```python
from build123d import *

# Parameters (mm, degrees)
EXTRUDE_1_DEPTH      = 20
EXTRUDE_1_DEPTH_BACK = 20
SKETCH_1_W           = 140
SKETCH_1_H           = 580
SKETCH_1_R           = 30
EXTRUDE_2_DEPTH      = 25
EXTRUDE_2_DEPTH_BACK = 65
SKETCH_3_R           = 30
CUT_EXTRUDE_1_DEPTH  = 40
FILLET_1_R           = 50
FILLET_2_R           = 15
CHAMFER_1_SIZE       = 20


with BuildPart() as part:
    # Эскиз1 → Бобышка-Вытянуть1 (new, two sides: drawn at the far end of the back side and taken through both)
    with BuildSketch(Plane.XY.offset(-EXTRUDE_1_DEPTH_BACK)):
        with Locations((0, -208.783389553)):
            Rectangle(SKETCH_1_W, SKETCH_1_H)
        with Locations((0, 41.216610447)):
            Circle(SKETCH_1_R, mode=Mode.SUBTRACT)
        with Locations((0, -458.783389553)):
            Circle(SKETCH_1_R, mode=Mode.SUBTRACT)
    extrude(amount=EXTRUDE_1_DEPTH + EXTRUDE_1_DEPTH_BACK)

    # Эскиз3 → Бобышка-Вытянуть2 (add, two sides: drawn at the far end of the back side and taken through both)
    with BuildSketch(Plane(origin=(0, 0, -20), x_dir=(-1, 0, 0), z_dir=(0, 0, -1)).offset(-EXTRUDE_2_DEPTH_BACK)):
        with Locations((0, 41.216610447)):
            Circle(SKETCH_3_R)
        with Locations((0, -458.783389553)):
            Circle(SKETCH_3_R)
    extrude(amount=EXTRUDE_2_DEPTH + EXTRUDE_2_DEPTH_BACK)

    # Эскиз4 → Вырез-Вытянуть1 (cut)
    with BuildSketch(Plane(origin=(0, 0, -20), x_dir=(-1, 0, 0), z_dir=(0, 0, -1))):
        Polygon((-30, 1.216610447), (0, 1.216610447), (30, 1.216610447), (30, -418.783389553), (0, -418.783389553), (-30, -418.783389553), align=None)
    extrude(amount=-CUT_EXTRUDE_1_DEPTH, mode=Mode.SUBTRACT)

    # Скругление1
    fillet_1_edges = [part.edges().sort_by_distance(p)[0] for p in [
        (70, -498.783389553, 0),
        (70, 81.216610447, 0),
        (-70, 81.216610447, 0),
        (-70, -498.783389553, 0),
    ]]
    fillet(fillet_1_edges, radius=FILLET_1_R)

    # Скругление2
    fillet_2_edges = [part.edges().sort_by_distance(p)[0] for p in [
        (30, 1.216610447, 0),
        (-30, 1.216610447, 0),
        (-30, -418.783389553, 0),
        (30, -418.783389553, 0),
    ]]
    fillet(fillet_2_edges, radius=FILLET_2_R)

    # Фаска1
    # the kernel refuses this chamfer: 20 mm, written as the material it takes off along each edge
    with BuildSketch(Plane(origin=(20, -498.783389553, -20), x_dir=(0, -0.0274958766105877, 0.9996219169112968), z_dir=(-1, 0, 0))) as chamfer_1_piece_1_section:
        Polygon((CHAMFER_1_SIZE * 0.999621916911, CHAMFER_1_SIZE * 0.0274958766106), (-CHAMFER_1_SIZE * 0.0274958766106, CHAMFER_1_SIZE * 0.999621916911), (0, 0), align=None)
    chamfer_1_piece_1 = extrude(amount=40, mode=Mode.PRIVATE)
    chamfer_1_piece_1 = chamfer_1_piece_1 - Plane(origin=(0, -458.783389553, -12.567480213), x_dir=(-1, 0, 0), z_dir=(0, 0, 1)) * Cylinder(30, 160, mode=Mode.PRIVATE)
    add(chamfer_1_piece_1, mode=Mode.SUBTRACT)
    with BuildSketch(Plane(origin=(-20, -448.783389553, -20), x_dir=(0, -1, 0), z_dir=(1, 0, 0))) as chamfer_1_piece_2_section:
        Polygon((50, -CHAMFER_1_SIZE), (50 - CHAMFER_1_SIZE, 0), (50, 0), align=None)
    chamfer_1_piece_2 = revolve(axis=Axis((-20, -448.783389553, -20), (0, 0, -1)), revolution_arc=90, mode=Mode.PRIVATE)
    chamfer_1_piece_2 = chamfer_1_piece_2 - Plane(origin=(0, -458.783389553, -13.088521936), x_dir=(-1, 0, 0), z_dir=(0, 0, 1)) * Cylinder(30, 200, mode=Mode.PRIVATE)
    add(chamfer_1_piece_2, mode=Mode.SUBTRACT)
    with BuildSketch(Plane(origin=(20, -448.783389553, -20), x_dir=(1, 0, 0), z_dir=(0, 1, 0))) as chamfer_1_piece_3_section:
        Polygon((50, -CHAMFER_1_SIZE), (50 - CHAMFER_1_SIZE, 0), (50, 0), align=None)
    chamfer_1_piece_3 = revolve(axis=Axis((20, -448.783389553, -20), (0, 0, -1)), revolution_arc=90, mode=Mode.PRIVATE)
    chamfer_1_piece_3 = chamfer_1_piece_3 - Plane(origin=(0, -458.783389553, -13.088521936), x_dir=(-1, 0, 0), z_dir=(0, 0, 1)) * Cylinder(30, 200, mode=Mode.PRIVATE)
    add(chamfer_1_piece_3, mode=Mode.SUBTRACT)
    with BuildSketch(Plane(origin=(-70, -448.783389553, -20), x_dir=(-0.027495876610586317, 0, 0.9996219169112968), z_dir=(0, 1, 0)), Plane(origin=(70, 31.216610447, -20), x_dir=(0.027495876610586317, 0, 0.9996219169112968), z_dir=(0, -1, 0)), Plane(origin=(70, 31.216610447, 20), x_dir=(-0.9996219169112968, 0, 0.027495876610586317), z_dir=(0, -1, 0)), Plane(origin=(-70, -448.783389553, 20), x_dir=(0.9996219169112968, 0, 0.027495876610586317), z_dir=(0, 1, 0))) as chamfer_1_piece_4:
        Polygon((CHAMFER_1_SIZE * 0.999621916911, CHAMFER_1_SIZE * 0.0274958766106), (-CHAMFER_1_SIZE * 0.0274958766106, CHAMFER_1_SIZE * 0.999621916911), (0, 0), align=None)
    extrude(amount=480, mode=Mode.SUBTRACT)
    with BuildSketch(Plane(origin=(-20, 31.216610447, -20), x_dir=(0, 1, 0), z_dir=(1, 0, 0))) as chamfer_1_piece_5_section:
        Polygon((50, CHAMFER_1_SIZE), (50 - CHAMFER_1_SIZE, 0), (50, 0), align=None)
    chamfer_1_piece_5 = revolve(axis=Axis((-20, 31.216610447, -20), (0, 0, 1)), revolution_arc=90, mode=Mode.PRIVATE)
    chamfer_1_piece_5 = chamfer_1_piece_5 - Plane(origin=(0, 41.216610447, -13.088521936), x_dir=(-1, 0, 0), z_dir=(0, 0, 1)) * Cylinder(30, 200, mode=Mode.PRIVATE)
    add(chamfer_1_piece_5, mode=Mode.SUBTRACT)
    with BuildSketch(Plane(origin=(20, 31.216610447, -20), x_dir=(1, 0, 0), z_dir=(0, -1, 0))) as chamfer_1_piece_6_section:
        Polygon((50, CHAMFER_1_SIZE), (50 - CHAMFER_1_SIZE, 0), (50, 0), align=None)
    chamfer_1_piece_6 = revolve(axis=Axis((20, 31.216610447, -20), (0, 0, 1)), revolution_arc=90, mode=Mode.PRIVATE)
    chamfer_1_piece_6 = chamfer_1_piece_6 - Plane(origin=(0, 41.216610447, -13.088521936), x_dir=(-1, 0, 0), z_dir=(0, 0, 1)) * Cylinder(30, 200, mode=Mode.PRIVATE)
    add(chamfer_1_piece_6, mode=Mode.SUBTRACT)
    with BuildSketch(Plane(origin=(-20, 81.216610447, -20), x_dir=(0, 0.027495876610586317, 0.9996219169112968), z_dir=(1, 0, 0))) as chamfer_1_piece_7_section:
        Polygon((CHAMFER_1_SIZE * 0.999621916911, CHAMFER_1_SIZE * 0.0274958766106), (-CHAMFER_1_SIZE * 0.0274958766106, CHAMFER_1_SIZE * 0.999621916911), (0, 0), align=None)
    chamfer_1_piece_7 = extrude(amount=40, mode=Mode.PRIVATE)
    chamfer_1_piece_7 = chamfer_1_piece_7 - Plane(origin=(0, 41.216610447, -12.567480213), x_dir=(-1, 0, 0), z_dir=(0, 0, 1)) * Cylinder(30, 160, mode=Mode.PRIVATE)
    add(chamfer_1_piece_7, mode=Mode.SUBTRACT)
    with BuildSketch(Plane(origin=(20, -498.783389553, 20), x_dir=(0, 0.9996219169112968, 0.027495876610586206), z_dir=(-1, 0, 0))) as chamfer_1_piece_8_section:
        Polygon((CHAMFER_1_SIZE * 0.999621916911, CHAMFER_1_SIZE * 0.0274958766106), (-CHAMFER_1_SIZE * 0.0274958766106, CHAMFER_1_SIZE * 0.999621916911), (0, 0), align=None)
    chamfer_1_piece_8 = extrude(amount=40, mode=Mode.PRIVATE)
    chamfer_1_piece_8 = chamfer_1_piece_8 - Plane(origin=(0, -458.783389553, 12.567480585), x_dir=(-1, 0, 0), z_dir=(0, 0, -1)) * Cylinder(30, 160, mode=Mode.PRIVATE)
    add(chamfer_1_piece_8, mode=Mode.SUBTRACT)
    with BuildSketch(Plane(origin=(20, -448.783389553, 20), x_dir=(1, 0, 0), z_dir=(0, 1, 0))) as chamfer_1_piece_9_section:
        Polygon((50 - CHAMFER_1_SIZE, 0), (50, CHAMFER_1_SIZE), (50, 0), align=None)
    chamfer_1_piece_9 = revolve(axis=Axis((20, -448.783389553, 20), (0, 0, -1)), revolution_arc=90, mode=Mode.PRIVATE)
    chamfer_1_piece_9 = chamfer_1_piece_9 - Plane(origin=(0, -458.783389553, 13.088521928), x_dir=(-1, 0, 0), z_dir=(0, 0, -1)) * Cylinder(30, 200, mode=Mode.PRIVATE)
    add(chamfer_1_piece_9, mode=Mode.SUBTRACT)
    with BuildSketch(Plane(origin=(-20, -448.783389553, 20), x_dir=(0, -1, 0), z_dir=(1, 0, 0))) as chamfer_1_piece_10_section:
        Polygon((50 - CHAMFER_1_SIZE, 0), (50, CHAMFER_1_SIZE), (50, 0), align=None)
    chamfer_1_piece_10 = revolve(axis=Axis((-20, -448.783389553, 20), (0, 0, -1)), revolution_arc=90, mode=Mode.PRIVATE)
    chamfer_1_piece_10 = chamfer_1_piece_10 - Plane(origin=(0, -458.783389553, 13.088521939), x_dir=(-1, 0, 0), z_dir=(0, 0, -1)) * Cylinder(30, 200, mode=Mode.PRIVATE)
    add(chamfer_1_piece_10, mode=Mode.SUBTRACT)
    with BuildSketch(Plane(origin=(20, 31.216610447, 20), x_dir=(1, 0, 0), z_dir=(0, -1, 0))) as chamfer_1_piece_11_section:
        Polygon((50 - CHAMFER_1_SIZE, 0), (50, -CHAMFER_1_SIZE), (50, 0), align=None)
    chamfer_1_piece_11 = revolve(axis=Axis((20, 31.216610447, 20), (0, 0, 1)), revolution_arc=90, mode=Mode.PRIVATE)
    chamfer_1_piece_11 = chamfer_1_piece_11 - Plane(origin=(0, 41.216610447, 13.088521931), x_dir=(-1, 0, 0), z_dir=(0, 0, -1)) * Cylinder(30, 200, mode=Mode.PRIVATE)
    add(chamfer_1_piece_11, mode=Mode.SUBTRACT)
    with BuildSketch(Plane(origin=(-20, 31.216610447, 20), x_dir=(0, 1, 0), z_dir=(1, 0, 0))) as chamfer_1_piece_12_section:
        Polygon((50 - CHAMFER_1_SIZE, 0), (50, -CHAMFER_1_SIZE), (50, 0), align=None)
    chamfer_1_piece_12 = revolve(axis=Axis((-20, 31.216610447, 20), (0, 0, 1)), revolution_arc=90, mode=Mode.PRIVATE)
    chamfer_1_piece_12 = chamfer_1_piece_12 - Plane(origin=(0, 41.216610447, 13.088521936), x_dir=(-1, 0, 0), z_dir=(0, 0, -1)) * Cylinder(30, 200, mode=Mode.PRIVATE)
    add(chamfer_1_piece_12, mode=Mode.SUBTRACT)
    with BuildSketch(Plane(origin=(-20, 81.216610447, 20), x_dir=(0, -0.9996219169112968, 0.027495876610586337), z_dir=(1, 0, 0))) as chamfer_1_piece_13_section:
        Polygon((CHAMFER_1_SIZE * 0.999621916911, CHAMFER_1_SIZE * 0.0274958766106), (-CHAMFER_1_SIZE * 0.0274958766106, CHAMFER_1_SIZE * 0.999621916911), (0, 0), align=None)
    chamfer_1_piece_13 = extrude(amount=40, mode=Mode.PRIVATE)
    chamfer_1_piece_13 = chamfer_1_piece_13 - Plane(origin=(0, 41.216610447, 12.567480585), x_dir=(-1, 0, 0), z_dir=(0, 0, -1)) * Cylinder(30, 160, mode=Mode.PRIVATE)
    add(chamfer_1_piece_13, mode=Mode.SUBTRACT)


solid = part.part
```
Verification items for the finished model (mm, model axes). A direction names the side the tool comes from. Coordinates: 2 decimals unless noted, no trailing zeros. Loops run counter-clockwise (first coordinate to the right, second up) from the corner with the lowest first, then second, coordinate; pieces in that order, holes last. Notation, with made-up numbers: (-20, 56) - (23, 56) arc R29 cw to (23, 76) - close; hole circle Ø7 at (67.5, 79). An arc over 180 degrees is marked (long way). Answer as a JSON object with one key per item and string values.
(1) Cross-section at B-B, the plane z = -36. Record the boundary of the cut face in (x, y).
Response:
{"outline": "circle Ø60 at (0, -458.78); circle Ø60 at (0, 41.22)"}
(2) Go/stop test with flat-tipped pins: pin 1 Ø12 at (x, z) = (-46, -8.5) entering from -Y; pin 2 Ø12 at (y, z) = (-240.5, 3.5) entering from +X; pin 3 Ø10 at (x, z) = (18, 33) entering from -Y. Record where each tip stops, or that it passes through.
Response:
{"pin 1": "stops at y = -489.44", "pin 2": "stops at x = 70", "pin 3": "stops at y = -485.82"}
(3) Scan lines: line 1 along Y through (x, z) = (0, -18); line 2 along Y through (x, z) = (-12, 7); line 3 along Z through (x, y) = (30.5, 55). Record each from-to range of solid material in increasing order.
Response:
{"line 1": "y = -488.78 to -418.78, 1.22 to 71.22", "line 2": "y = -491.78 to -418.78, 1.22 to 74.22", "line 3": "z = -20 to 20"}
(4) Cross-section at A-A, the plane x = 0. Record the boundary of the cut face in (y, z).
Response:
{"outline": "(-498.78, 0) - (-488.78, -10) - (-488.78, -45) - (-428.78, -45) - (-428.78, -20) - (-418.78, -20) - (-418.78, 20) - (-428.78, 20) - (-428.78, 45) - (-488.78, 45) - (-488.78, 10) - close; (1.22, -20) - (11.22, -20) - (11.22, -45) - (71.22, -45) - (71.22, -10) - (81.22, 0) - (71.22, 10) - (71.22, 45) - (11.22, 45) - (11.22, 20) - (1.22, 20) - close"}
(5) Mould release check, pull along X, two halves, no side actions. Record for faces 1 (the cylindrical face through (-25.723, -414.273, 0.28)), 2 (the cylindrical face through (25.489, -414.506, 0.28)), 3 (the flat face through (0.28, -491.8, 6.983)), 4 (the cylindrical face through (3.91, 70.96, 31.19)): pulls with the +X half, pulls with the -X half, needs draft (parallel to the pull), parting line crosses it, or undercut.
Response:
{"face 1": "undercut", "face 2": "undercut", "face 3": "needs draft", "face 4": "parting line crosses it"}
(6) Access from +Z, -Z, +X, -X, +Y, -Y to the whole of each face (thin tool, end or side, straight path). Record for faces 5 (the cylindrical face through (25.72, -3.29, 0.28)), 6 (the flat face through (0, -458, 45)), 7 (the cylindrical face through (-13.84, -485.4, -30.68)).
Response:
{"face 5": "+Z, -Z", "face 6": "+Z, +X, -X, +Y, -Y", "face 7": "-Z"}
